```python
from build123d import *

# Parameters (mm, degrees)
SKETCH1_R           = 2.875
SKETCH1_R_2         = 1.925
BOSS_EXTRUDE1_DEPTH = 2
SKETCH2_R           = 1.925
SKETCH2_R_2         = 2.875
BOSS_EXTRUDE2_DEPTH = 1.45
SKETCH3_R           = 2.75
SKETCH3_R_2         = 2.1
BOSS_EXTRUDE3_DEPTH = 0.7
CUT_EXTRUDE1_START  = -1.3
SKETCH5_R           = 2.1
CUT_EXTRUDE1_DEPTH  = 1.3
SKETCH6_R           = 0.85
CUT_EXTRUDE2_DEPTH  = 18.033900023
SKETCH7_R           = 0.45
CUT_EXTRUDE3_DEPTH  = 18.144496201
SKETCH8_R           = 1.925
CUT_EXTRUDE4_DEPTH  = 0.75


with BuildPart() as part:
    # Sketch1 → Boss-Extrude1 (new body)
    with BuildSketch(Plane(origin=(0, 0, 0), x_dir=(1, 0, 0), z_dir=(0, 1, 0))):
        with Locations(Location((0, 0, 0), (0, 0, 270))):
            Circle(SKETCH1_R)
        with Locations(Location((0, 0, 0), (0, 0, 270))):
            Circle(SKETCH1_R_2, mode=Mode.SUBTRACT)
    extrude(amount=BOSS_EXTRUDE1_DEPTH)

    # Sketch2 → Boss-Extrude2 (add)
    # profile 1 of 7: a face of its own
    with BuildSketch(Plane(origin=(0, 2, 0), x_dir=(1, 0, 0), z_dir=(0, 1, 0))):
        with Locations((-9.95, 0)):
            Circle(SKETCH2_R)
    # profile 2 of 7: a face of its own
    with BuildSketch(Plane(origin=(0, 2, 0), x_dir=(1, 0, 0), z_dir=(0, 1, 0))):
        with BuildLine():
            ThreePointArc((1.925, 9.95), (-0.129680261, 8.029373011), (-1.907527823, 10.208771335))
            Line((-1.907527823, 10.208771335), (-2.899137803, 2.899137803))
            Line((-2.899137803, 2.899137803), (-10.208771335, 1.907527823))
            ThreePointArc((-10.208771335, 1.907527823), (-8.683609424, 1.44978616), (-8.025, 0))
            ThreePointArc((-8.025, 0), (-8.683609424, -1.44978616), (-10.208771335, -1.907527823))
            Line((-10.208771335, -1.907527823), (-2.899137803, -2.899137803))
            Line((-2.899137803, -2.899137803), (-1.907527823, -10.208771335))
            ThreePointArc((-1.907527823, -10.208771335), (-0.129680261, -8.029373011), (1.925, -9.95))
            ThreePointArc((1.925, -9.95), (1.920626989, -10.079680261), (1.907527823, -10.208771335))
            Line((1.907527823, -10.208771335), (2.899137803, -2.899137803))
            Line((2.899137803, -2.899137803), (10.208771335, -1.907527823))
            ThreePointArc((10.208771335, -1.907527823), (8.025, 0), (10.208771335, 1.907527823))
            Line((10.208771335, 1.907527823), (2.899137803, 2.899137803))
            Line((2.899137803, 2.899137803), (1.907527823, 10.208771335))
            ThreePointArc((1.907527823, 10.208771335), (1.920626989, 10.079680261), (1.925, 9.95))
        make_face()
        with Locations(Location((0, 0, 0), (0, 0, 270))):
            Circle(SKETCH2_R_2, mode=Mode.SUBTRACT)
    # profile 3 of 7: a face of its own
    with BuildSketch(Plane(origin=(0, 2, 0), x_dir=(1, 0, 0), z_dir=(0, 1, 0))):
        with Locations(Location((0, 0, 0), (0, 0, 270))):
            Circle(SKETCH2_R_2)
        with Locations(Location((0, 0, 0), (0, 0, 270))):
            Circle(SKETCH2_R, mode=Mode.SUBTRACT)
    # profile 4 of 7: a face of its own
    with BuildSketch(Plane(origin=(0, 2, 0), x_dir=(1, 0, 0), z_dir=(0, 1, 0))):
        with Locations(Location((0, 0, 0), (0, 0, 270))):
            Circle(SKETCH2_R)
    # profile 5 of 7: a face of its own
    with BuildSketch(Plane(origin=(0, 2, 0), x_dir=(1, 0, 0), z_dir=(0, 1, 0))):
        with Locations((0, -9.95)):
            Circle(SKETCH2_R)
    # profile 6 of 7: a face of its own
    with BuildSketch(Plane(origin=(0, 2, 0), x_dir=(1, 0, 0), z_dir=(0, 1, 0))):
        with Locations((9.95, 0)):
            Circle(SKETCH2_R)
    # profile 7 of 7: a face of its own
    with BuildSketch(Plane(origin=(0, 2, 0), x_dir=(1, 0, 0), z_dir=(0, 1, 0))):
        with Locations((0, 9.95)):
            Circle(SKETCH2_R)
    extrude(amount=BOSS_EXTRUDE2_DEPTH)

    # Sketch3 → Boss-Extrude3 (add)
    with BuildSketch(Plane(origin=(0, 3.45, 0), x_dir=(1, 0, 0), z_dir=(0, 1, 0))):
        with Locations(Location((0, 0, 0), (0, 0, 270))):
            Circle(SKETCH3_R)
        with Locations(Location((0, 0, 0), (0, 0, 270))):
            Circle(SKETCH3_R_2, mode=Mode.SUBTRACT)
    extrude(amount=BOSS_EXTRUDE3_DEPTH)

    # Sketch5 → Cut-Extrude1 (cut)
    with BuildSketch(Plane(origin=(0, 4.15, 0), x_dir=(1, 0, 0), z_dir=(0, 1, 0)).offset(CUT_EXTRUDE1_START)):
        with Locations(Location((0, 0, 0), (0, 0, 270))):
            Circle(SKETCH5_R)
    extrude(amount=CUT_EXTRUDE1_DEPTH, mode=Mode.SUBTRACT)

    # Sketch6 → Cut-Extrude2 (cut, through all)
    with BuildSketch(Plane(origin=(0, 2.85, 0), x_dir=(1, 0, 0), z_dir=(0, 1, 0))):
        with Locations(Location((0, 0, 0), (0, 0, 270))):
            Circle(SKETCH6_R)
    extrude(amount=-CUT_EXTRUDE2_DEPTH, mode=Mode.SUBTRACT)

    # Sketch7 → Cut-Extrude3 (cut, through all)
    with BuildSketch(Plane(origin=(0, 3.45, 0), x_dir=(1, 0, 0), z_dir=(0, 1, 0))):
        with Locations(Location((0, 10.025, 0), (0, 0, 270))):
            Circle(SKETCH7_R)
        with Locations(Location((0, 6.525, 0), (0, 0, 270))):
            Circle(SKETCH7_R)
        with Locations(Location((6.525, 0, 0), (0, 0, 270))):
            Circle(SKETCH7_R)
        with Locations(Location((10.025, 0, 0), (0, 0, 270))):
            Circle(SKETCH7_R)
        with Locations(Location((0, -6.525, 0), (0, 0, 270))):
            Circle(SKETCH7_R)
        with Locations(Location((0, -10.025, 0), (0, 0, 270))):
            Circle(SKETCH7_R)
        with Locations(Location((-6.525, 0, 0), (0, 0, 270))):
            Circle(SKETCH7_R)
        with Locations(Location((-10.025, 0, 0), (0, 0, 270))):
            Circle(SKETCH7_R)
    extrude(amount=-CUT_EXTRUDE3_DEPTH, mode=Mode.SUBTRACT)

    # Sketch8 → Cut-Extrude4 (cut)
    with BuildSketch(Plane.XZ.offset(-2)):
        with Locations(Location((0, 0, 0), (0, 0, 270))):
            Circle(SKETCH8_R)
    extrude(amount=-CUT_EXTRUDE4_DEPTH, mode=Mode.SUBTRACT)


solid = part.part
```
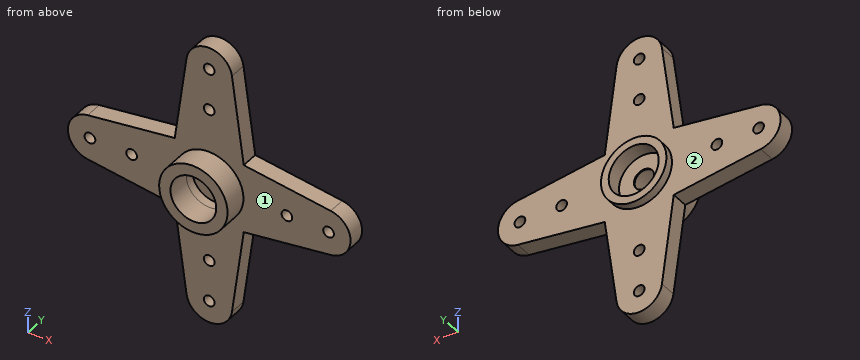
Work out the finished part from the listing and answer in its coordinate system (mm). Face numbers are marked on the shaded views. A direction names the side the tool comes from. Round coordinates to 2 decimals unless told otherwise and drop trailing zeros. Write each loop counter-clockwise with the first axis right and the second up, starting at its lowest first coordinate (ties: lowest second). Pieces come first, ordered by that corner, then holes.
1) Flat-ended cylindrical pins translate along their axes: P1, Ø3, axis at x = 0, z = 0, coming from the +Y side; P2, Ø2.5, axis at x = 0, z = 0, coming from the -Y side; P3, Ø3, axis at x = 3.5, z = 5.5, coming from the -Y side. Find the tip coordinate at first contact, or state that the pin passes through.
2) A cutting plane is placed at D-D on x = 3.25. Determine the outline of the cut face in (y, z).
3) A cutting plane is placed at A-A on y = 1.7. Determine the outline of the cut face in (x, z) (3 decimals).
4) A cutting plane is placed at B-B on z = 0. Give the number of separate pieces and of enclosed holes in the cut face, and give its area (4 significant figures).
5) Which of the six approach directions +Z, -Z, +X, -X, +Y, -Y give full straight-line access (tool end or side, diameter ignored) to the marked faces 1 and 2?
6) Consider probe 1 along X at (y, z) = (2.6, 0) (3 decimals); probe 2 along X at (y, z) = (3, 0) (3 decimals); probe 3 along Y at (x, z) = (-7.25, 2.25). Determine where each line is inside the solid, lowest interval first.
Entries:
1. P1: stops at y = 2.85
1. P2: stops at y = 2.75
1. P3: stops at y = 2
2. outline: (2, -2.85) - (3.45, -2.85) - (3.45, 2.85) - (2, 2.85) - close
3. outline: circle Ø5.75 at (0, 0); hole circle Ø3.85 at (0, 0)
4. separate pieces: 6
4. enclosed holes: 0
4. area: 28.35 mm2
5. face 1: -Y
5. face 2: +Y
6. probe 1: x = -11.875 to -10.475, -9.575 to -6.975, -6.075 to -1.925, 1.925 to 6.075, 6.975 to 9.575, 10.475 to 11.875
6. probe 2: x = -11.875 to -10.475, -9.575 to -6.975, -6.075 to -2.1, 2.1 to 6.075, 6.975 to 9.575, 10.475 to 11.875
6. probe 3: y = 2 to 3.45
